```python
from build123d import *

# Parameters (mm, degrees)
SKETCH_1_R          = 40
SKETCH_1_R_2        = 2.1
EXTRUDE_1_DEPTH     = 5
SKETCH_2_R          = 3.05
CUT_EXTRUDE_2_DEPTH = 10


with BuildPart() as part:
    # 草图1 → 凸台-拉伸1 (new body)
    with BuildSketch(Plane.XY):
        Circle(SKETCH_1_R)
        with Locations((14.938938215, 8.625)):
            Circle(SKETCH_1_R_2, mode=Mode.SUBTRACT)
        with Locations((14.938938215, -8.625)):
            Circle(SKETCH_1_R_2, mode=Mode.SUBTRACT)
        with Locations((0, -17.25)):
            Circle(SKETCH_1_R_2, mode=Mode.SUBTRACT)
        with Locations((-14.938938215, -8.625)):
            Circle(SKETCH_1_R_2, mode=Mode.SUBTRACT)
        with Locations((-14.938938215, 8.625)):
            Circle(SKETCH_1_R_2, mode=Mode.SUBTRACT)
    extrude(amount=EXTRUDE_1_DEPTH)

    # 草图2 → 切除-拉伸2 (cut)
    with BuildSketch(Plane.XY.offset(5)):
        with Locations((0, 30)):
            Circle(SKETCH_2_R)
    extrude(amount=-CUT_EXTRUDE_2_DEPTH, mode=Mode.SUBTRACT)


solid = part.part
```
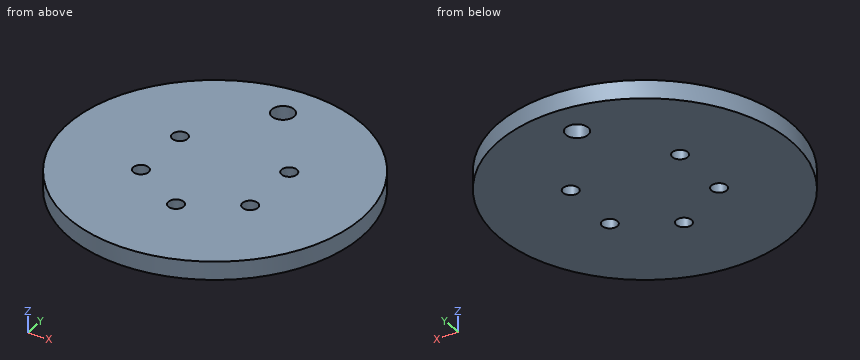
Can you work these out from the model? Positions are in its coordinate system, mm. Coordinates: 2 decimals unless noted, no trailing zeros. Loops run counter-clockwise (first coordinate to the right, second up) from the corner with the lowest first, then second, coordinate; pieces in that order, holes last. Notation, with made-up numbers: (52.5, 14.25) -> (104.5, 14.25) arc R14 cw to (104.5, 28.25) -> close; hole circle Ø5 at (79.25, -12). An arc over 180 degrees is marked (long way). Answer as a JSON object with one key per item and string values.
1) Imagine slicing it at C-C (z = 3.5). Please give me the cut outline in (x, y) (3 decimals), then the cut area to 3 significant figures.
Results:
{"outline": "circle Ø80 at (0, 0); hole circle Ø4.2 at (-14.939, -8.625); hole circle Ø4.2 at (-14.939, 8.625); hole circle Ø6.1 at (0, 30); hole circle Ø4.2 at (0, -17.25); hole circle Ø4.2 at (14.939, -8.625); hole circle Ø4.2 at (14.939, 8.625)", "area": "4,930 mm^2"}
2) Imagine slicing it at B-B (y = 30). Please give me the cut outline in (x, z).
Results:
{"outline": "(-26.46, 0) -> (-3.05, 0) -> (-3.05, 5) -> (-26.46, 5) -> close; (3.05, 0) -> (26.46, 0) -> (26.46, 5) -> (3.05, 5) -> close"}
3) Imagine slicing it at A-A (x = 0). Please give me the cut outline in (y, z), then the cut area to 4 significant figures.
Results:
{"outline": "(-40, 0) -> (-19.35, 0) -> (-19.35, 5) -> (-40, 5) -> close; (-15.15, 0) -> (26.95, 0) -> (26.95, 5) -> (-15.15, 5) -> close; (33.05, 0) -> (40, 0) -> (40, 5) -> (33.05, 5) -> close", "area": "348.5 mm^2"}
4) If I drill on line 1 (Y direction, x = 0, z = 1.45); line 2 (X direction, y = 9.5, z = 3.1); line 3 (X direction, y = 32, z = 4.75), over which ranges is the centre line in solid material (lowest first)?
Results:
{"line 1": "y = -40 to -19.35, -15.15 to 26.95, 33.05 to 40", "line 2": "x = -38.86 to -16.85, -13.03 to 13.03, 16.85 to 38.86", "line 3": "x = -24 to -2.3, 2.3 to 24"}
5) Imagine slicing it at D-D (y = -17.25). Please give me the cut outline in (x, z), then the cut area to 3 significant figures.
Results:
{"outline": "(-36.09, 0) -> (-2.1, 0) -> (-2.1, 5) -> (-36.09, 5) -> close; (2.1, 0) -> (36.09, 0) -> (36.09, 5) -> (2.1, 5) -> close", "area": "340 mm^2"}
6) For P1, Ø3.5, axis at x = 0, y = 30, coming from the +Z side, with a flat end and sliding along its axis, tell me the tip position at first contact or that it passes through.
Results:
{"P1": "passes through"}
